Geometry: final body of the model. Coordinates: model frame, mm. A direction names the side the tool comes from. Give positions to 0.01 mm unless a question says otherwise; leave off trailing zeros. Loops run counter-clockwise (first coordinate to the right, second up) from the corner with the lowest first, then second, coordinate; pieces in that order, holes last. Notation, with made-up numbers: (4, 21) - (12, 21) arc R20 cw to (12, 51) - close; hole circle Ø11 at (17, 55.25). An arc over 180 degrees is marked (long way). Answer in a Markdown table with one row per item.
from build123d import *

# Parameters (mm, degrees)
MODEL_R             = 6
MODEL_R_2           = 5
MODEL_R_3           = 4
MODEL_W             = 10
MODEL_H             = 12.4
BOSS_EXTRUDE1_DEPTH = 12.4


with BuildPart() as part:
    # Model → Boss-Extrude1 (new body)
    with BuildSketch(Plane.XY):
        with BuildLine():
            Line((-27.5, 0), (0, 0))
            Line((0, 0), (0, 190))
            Line((0, 190), (-27.5, 190))
            ThreePointArc((-27.5, 190), (-29.267766953, 189.267766953), (-30, 187.5))
            Line((-30, 187.5), (-30, 2.5))
            ThreePointArc((-30, 2.5), (-29.267766953, 0.732233047), (-27.5, 0))
        make_face()
        with Locations(Location((-15, 165, 0), (0, 0, 180))):
            Circle(MODEL_R, mode=Mode.SUBTRACT)
        with Locations(Location((-15, 95, 0), (0, 0, 180))):
            Circle(MODEL_R_2, mode=Mode.SUBTRACT)
        with Locations(Location((-15, 115, 0), (0, 0, 180))):
            Circle(MODEL_R_3, mode=Mode.SUBTRACT)
        with Locations(Location((-15, 25, 0), (0, 0, 180))):
            Circle(MODEL_R, mode=Mode.SUBTRACT)
        with Locations(Location((-15, 75, 0), (0, 0, 180))):
            Circle(MODEL_R_3, mode=Mode.SUBTRACT)
        with Locations((-15, 136.2)):
            Rectangle(MODEL_W, MODEL_H, mode=Mode.SUBTRACT)
        with Locations((-15, 53.8)):
            Rectangle(MODEL_W, MODEL_H, mode=Mode.SUBTRACT)
    extrude(amount=BOSS_EXTRUDE1_DEPTH)


solid = part.part
Q1. First-contact query: pin 1 (5 mm diameter, centred on x = -15, y = 115, fed in from +Z). Flat tip, straight axial feed; report the tip coordinate or a pass-through.
Check values:
| item | result |
|---|---|
| pin 1 | through |
Q2. Cut plane A-A (y = 165). Output: boundary loops of the cut face in (x, z).
Check values:
| item | result |
|---|---|
| outline | (-30, 0) - (-21, 0) - (-21, 12.4) - (-30, 12.4) - close; (-9, 0) - (0, 0) - (0, 12.4) - (-9, 12.4) - close |
Q3. Cut plane D-D (y = 115). Output: boundary loops of the cut face in (x, z).
Check values:
| item | result |
|---|---|
| outline | (-30, 0) - (-19, 0) - (-19, 12.4) - (-30, 12.4) - close; (-11, 0) - (0, 0) - (0, 12.4) - (-11, 12.4) - close |
Q4. Draft query along X for faces 3 (the flat face through (-14, 0, 6)), 4 (the cylindrical face through (-17.769, 170.323, 6.113)), 5 (the flat face through (0, 94, 6)). Return one class per face: pulls with the +X half, pulls with the -X half, needs draft (parallel to the pull), parting line crosses it, or undercut.
Check values:
| item | result |
|---|---|
| face 3 | needs draft |
| face 4 | undercut |
| face 5 | pulls with the +X half |
Q5. Material intervals for line 1 along X through (y, z) = (165, 8.75); line 2 along X through (y, z) = (20.5, 10.75), sorted ascending.
Check values:
| item | result |
|---|---|
| line 1 | -30 to -21, -9 to 0 |
| line 2 | -30 to -18.97, -11.03 to 0 |
Q6. Reachability of faces 1 (the flat face through (-14, 190, 6)), 2 (the flat face through (-10, 54, 6)) from +Z, -Z, +X, -X, +Y, -Y: full face, straight path, thin tool, end or side. Return the list, or none.
Check values:
| item | result |
|---|---|
| face 1 | +Z, -Z, +X, -X, +Y |
| face 2 | +Z, -Z |
Q7. Cut plane B-B (x = -15). Give the number of separate pieces and of enclosed holes in the cut face, and give its area (3 significant figures).
Check values:
| item | result |
|---|---|
| separate pieces | 8 |
| enclosed holes | 0 |
| area | 1,430 mm² |
Q8. Cut plane C-C (z = 4.75). Output: boundary loops of the cut face in (x, y).
Check values:
| item | result |
|---|---|
| outline | (-30, 2.5) arc R2.5 ccw to (-27.5, 0) - (0, 0) - (0, 190) - (-27.5, 190) arc R2.5 ccw to (-30, 187.5) - close; hole circle Ø12 at (-15, 25); hole circle Ø12 at (-15, 165); hole (-20, 47.6) - (-10, 47.6) - (-10, 60) - (-20, 60) - close; hole circle Ø10 at (-15, 95); hole (-20, 130) - (-10, 130) - (-10, 142.4) - (-20, 142.4) - close; hole circle Ø8 at (-15, 75); hole circle Ø8 at (-15, 115) |
